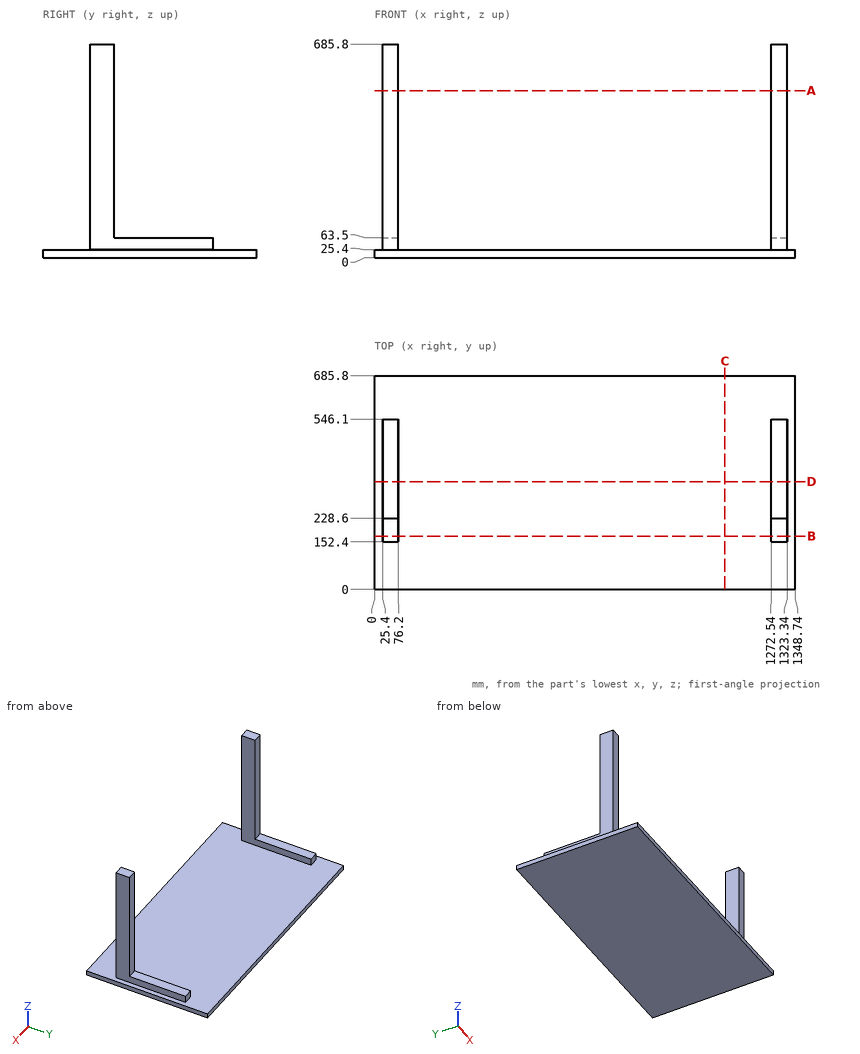
For this review, use the dimensioned drawing (mm, ordinates from the lowest corner) and the shaded views. Give positions to 0.01 mm unless a question says otherwise; leave off trailing zeros. Order: outer loops, then holes, each group sorted by start corner. A loop starts at its lowest first (then second) coordinate and runs counter-clockwise, first axis right, second up. Notation, with made-up numbers: (-38.5, 10) - (-32.5, 10) arc R36 cw to (-32.5, 49) - close; hole circle Ø5 at (-10, -11.75). An arc over 180 degrees is marked (long way). Use CSV: the item, a comma, the result in double quotes. Start each with the question number.
Q1. For line 1 (X direction, y = 167, z = 455); line 2 (Z direction, x = 279, y = 293); line 3 (Z direction, x = 70, y = 262.5), list the stretches that pass through material, from the lowest coordinate up.
Q2. Take a section at C-C (x = 1124). State the section outline as (y, z) points, and give its area (3 significant figures).
Q3. Take a section at B-B (y = 171). State the section outline as (x, z) points.
Q4. For P1, Ø1, axis at y = 158.5, z = 79.5, coming from the +X side; P2, Ø15, axis at x = 43.5, z = 458.5, coming from the -Y side; P3, Ø3, axis at x = 227.5, y = 449, coming from the -Z side; P4, Ø12, axis at y = 222.5, z = 346.5, coming from the -X side, all flat-tipped, find the tip position at first contact; note any pin that passes through.
Q5. Take a section at A-A (z = 536). State the section outline as (x, y) points, and give its area (3 significant figures).
Q6. Take a section at D-D (y = 346). State the section outline as (x, z) points.
Calculated:
1,line 1,"x = 25.4 to 76.2, 1272.54 to 1323.34"
1,line 2,"z = 0 to 25.4"
1,line 3,"z = 0 to 63.5"
2,outline,"(0, 0) - (685.8, 0) - (685.8, 25.4) - (0, 25.4) - close"
2,area,"17,400 mm²"
3,outline,"(0, 0) - (1348.74, 0) - (1348.74, 25.4) - (1323.34, 25.4) - (1323.34, 685.8) - (1272.54, 685.8) - (1272.54, 25.4) - (76.2, 25.4) - (76.2, 685.8) - (25.4, 685.8) - (25.4, 25.4) - (0, 25.4) - close"
4,P1,"stops at x = 1323.34"
4,P2,"stops at y = 152.4"
4,P3,"stops at z = 0"
4,P4,"stops at x = 25.4"
5,outline,"(25.4, 152.4) - (76.2, 152.4) - (76.2, 228.6) - (25.4, 228.6) - close; (1272.54, 152.4) - (1323.34, 152.4) - (1323.34, 228.6) - (1272.54, 228.6) - close"
5,area,"7,740 mm²"
6,outline,"(0, 0) - (1348.74, 0) - (1348.74, 25.4) - (1323.34, 25.4) - (1323.34, 63.5) - (1272.54, 63.5) - (1272.54, 25.4) - (76.2, 25.4) - (76.2, 63.5) - (25.4, 63.5) - (25.4, 25.4) - (0, 25.4) - close"
